Check sheet for the modelled part. Datum: model origin and axes. Units: mm. A direction names the side the tool comes from. Give positions to 0.01 mm unless a question says otherwise; leave off trailing zeros. Answer in a Markdown table with one row per item. Add a question column.
(1) Go/stop test with a flat-tipped pin: pin 1 (4 mm diameter, centred on x = 23.5, y = -7.5, fed in from -Z). Record where the tip stops, or that it passes through.
(2) Thickness scan on L1, parallel to X at y = -6, z = 15.5; L2, parallel to Y at x = 27, z = 37; L3, parallel to X at y = -11.5, z = 26. Record the ranges inside material, lowest first. Write a range as [from, to].
(3) Release check for a two-part mould opening along Y. For faces 1 (the face through (29.176, -9.254, 4.93)), 2 (the face through (5, -33.052, 20)), 3 (the face through (55.36, -8, 20)), 4 (the face through (5, 16.948, 20)) record: released by +Y, released by -Y, zero draft, split by the parting line, or undercut.
(4) Set-up check for faces 5 (the face through (5, -8, 40)), 6 (the face through (27, -11, 10)), 7 (the face through (21.665, -9.584, 24.93)): record each of +Z, -Z, +X, -X, +Y, -Y from which the full face is reachable in a straight line by a thin tool's end or side.
```python
from build123d import *

# Parameters (mm, degrees)
F0_W           = 100
F0_H           = 50
F1_DEPTH       = 40
F3_D           = 8
F3_DEPTH       = 20
F3_CBORE_D     = 10
F3_CBORE_DEPTH = 10
F3_TIP         = 2.4034424761
F5_D           = 6
F5_DEPTH       = 20
F5_CBORE_D     = 8
F5_CBORE_DEPTH = 10
F5_TIP         = 1.8025818571


with BuildPart() as f1:
    # F0 (on Top) → F1 (new body)
    with BuildSketch(Plane.XY):
        with Locations((5.3602904081, -8.052177819)):
            Rectangle(F0_W, F0_H)
    extrude(amount=F1_DEPTH)

    # F3
    with Locations(Plane.XY.offset(40)):
        with Locations((25.3602904081, -8.052177819)):
            CounterBoreHole(F3_D / 2, F3_CBORE_D / 2, F3_CBORE_DEPTH, depth=F3_DEPTH)
            with Locations((0, 0, -(F3_DEPTH + F3_TIP / 2))):  # 118° drill point
                Cone(0, F3_D / 2, F3_TIP, mode=Mode.SUBTRACT)

    # F5
    with Locations(Plane(origin=(0, 0, 0), x_dir=(1, 0, 0), z_dir=(0, 0, -1))):
        with Locations((25.3602904081, 8.052177819)):
            CounterBoreHole(F5_D / 2, F5_CBORE_D / 2, F5_CBORE_DEPTH, depth=F5_DEPTH)
            with Locations((0, 0, -(F5_DEPTH + F5_TIP / 2))):  # 118° drill point
                Cone(0, F5_D / 2, F5_TIP, mode=Mode.SUBTRACT)


solid = f1.part
```
Answer below:
| question | item | result |
|---|---|---|
| 1 | pin 1 | stops at z = 10 |
| 2 | L1 | x = [-44.64, 23.17], [27.55, 55.36] |
| 2 | L2 | y = [-33.05, -12.78], [-3.33, 16.95] |
| 2 | L3 | x = [-44.64, 23.33], [27.39, 55.36] |
| 3 | face 1 | undercut |
| 3 | face 2 | released by -Y |
| 3 | face 3 | zero draft |
| 3 | face 4 | released by +Y |
| 4 | face 5 | +Z, +X, -X, +Y, -Y |
| 4 | face 6 | -Z |
| 4 | face 7 | +Z |
